Model file for the job. Use its own axes, mm. Give positions to 0.01 mm unless a question says otherwise; leave off trailing zeros. Order: outer loops, then holes, each group sorted by start corner. A loop starts at its lowest first (then second) coordinate and runs counter-clockwise, first axis right, second up. Notation, with made-up numbers: M 63,-33.5 L 108,-33.5 A25 ccw 108,-6.5 Z; hole C -7.5,73 d10. An arc over 180 degrees is marked long. Return JSON: item names as keys, results as strings. Group by question number.
1. Pin check, flat tip, straight feed: pin 1 (3 mm diameter, centred on x = -50, y = 50, fed in from +Z). Stop position of the tip, or through.
2. Slice it at B-B on z = -0.35. Give the number of separate pieces and of enclosed holes in the cut face, then the cut area to 3 significant figures.
3. Wall check: probe 1 along X at (y, z) = (-7, -0.2) (3 decimals); probe 2 along X at (y, z) = (-40, -0.9) (3 decimals); probe 3 along Y at (x, z) = (-50, -0.8) (3 decimals). Give the ranges that are in metal, low to high. Write a range as [from, to].
4. Slice it at A-A on y = 8.5. List the corners of the cut face in (x, z) (3 decimals), then the cut area to 4 significant figures.
from build123d import *

# Parameters (mm, degrees)
PAD_DEPTH        = 1
POCKET_DEPTH     = 0.001
HOLE_D           = 1.75
HOLE_CSINK_D     = 3.3
HOLE_CSINK_ANGLE = 90
SKETCH007_R      = 4.9
HOLE005_DEPTH    = 1.001
SKETCH008_R      = 1.5
HOLE006_DEPTH    = 1.001
SKETCH009_R      = 4.9
HOLE007_DEPTH    = 1.001
SKETCH010_R      = 1.5
HOLE008_DEPTH    = 1.001
POCKET001_DEPTH  = 1.001
SKETCH012_R      = 1.5
HOLE009_DEPTH    = 1.001


with BuildPart() as part:
    # Sketch → Pad (new body)
    with BuildSketch(Plane.XY):
        with BuildLine():
            Line((-51.8, 52.175), (51.8, 52.175))
            ThreePointArc((52.175, 51.8), (52.065165, 52.065165), (51.8, 52.175))
            Line((52.175, 51.8), (52.175, -51.8))
            ThreePointArc((51.8, -52.175), (52.065165, -52.065165), (52.175, -51.8))
            Line((51.8, -52.175), (-51.8, -52.175))
            ThreePointArc((-52.175, -51.8), (-52.065165, -52.065165), (-51.8, -52.175))
            Line((-52.175, -51.8), (-52.175, 51.8))
            ThreePointArc((-51.8, 52.175), (-52.065165, 52.065165), (-52.175, 51.8))
        make_face()
    extrude(amount=-PAD_DEPTH)

    # Sketch002 → Pocket (cut, through all)
    with BuildSketch(Plane.XY.offset(-4.8)):
        with BuildLine():
            Line((-45, 50.175), (45, 50.175))
            ThreePointArc((45, 50.175), (45.353553, 50.321447), (45.5, 50.675))
            ThreePointArc((45.5, 50.675), (45.353553, 51.028553), (45, 51.175))
            Line((-45, 51.175), (45, 51.175))
            ThreePointArc((-45, 51.175), (-45.353553, 51.028553), (-45.5, 50.675))
            ThreePointArc((-45.5, 50.675), (-45.353553, 50.321447), (-45, 50.175))
        make_face()
        with BuildLine():
            Line((-45, -51.175), (45, -51.175))
            ThreePointArc((45, -51.175), (45.353553, -51.028553), (45.5, -50.675))
            ThreePointArc((45.5, -50.675), (45.353553, -50.321447), (45, -50.175))
            Line((-45, -50.175), (45, -50.175))
            ThreePointArc((-45, -50.175), (-45.353553, -50.321447), (-45.5, -50.675))
            ThreePointArc((-45.5, -50.675), (-45.353553, -51.028553), (-45, -51.175))
        make_face()
        with BuildLine():
            Line((51.175, -45), (51.175, 45))
            ThreePointArc((51.175, 45), (51.028553, 45.353553), (50.675, 45.5))
            ThreePointArc((50.675, 45.5), (50.321447, 45.353553), (50.175, 45))
            Line((50.175, -45), (50.175, 45))
            ThreePointArc((50.175, -45), (50.321447, -45.353553), (50.675, -45.5))
            ThreePointArc((50.675, -45.5), (51.028553, -45.353553), (51.175, -45))
        make_face()
        with BuildLine():
            Line((-50.175, -45), (-50.175, 45))
            ThreePointArc((-50.175, 45), (-50.321447, 45.353553), (-50.675, 45.5))
            ThreePointArc((-50.675, 45.5), (-51.028553, 45.353553), (-51.175, 45))
            Line((-51.175, -45), (-51.175, 45))
            ThreePointArc((-51.175, -45), (-51.028553, -45.353553), (-50.675, -45.5))
            ThreePointArc((-50.675, -45.5), (-50.321447, -45.353553), (-50.175, -45))
        make_face()
    extrude(amount=-POCKET_DEPTH, mode=Mode.SUBTRACT)

    # Hole (through all)
    with Locations(Plane.XY):
        with Locations((-50, 50), (50, 50), (50, -50), (-50, -50)):
            CounterSinkHole(HOLE_D / 2, HOLE_CSINK_D / 2, counter_sink_angle=HOLE_CSINK_ANGLE)

    # Sketch007 → Hole005 (cut, through all)
    with BuildSketch(Plane.XY):
        with Locations((-40.005, -40.005)):
            Circle(SKETCH007_R)
        with Locations((-13.335, -40.005)):
            Circle(SKETCH007_R)
        with Locations((13.335, -40.005)):
            Circle(SKETCH007_R)
        with Locations((40.005, -40.005)):
            Circle(SKETCH007_R)
    extrude(amount=-HOLE005_DEPTH, mode=Mode.SUBTRACT)

    # Sketch008 → Hole006 (cut, through all)
    with BuildSketch(Plane.XY):
        with Locations((-40.005, -31.505)):
            Circle(SKETCH008_R)
        with Locations((-13.335, -31.505)):
            Circle(SKETCH008_R)
        with Locations((13.335, -31.505)):
            Circle(SKETCH008_R)
        with Locations((40.005, -31.505)):
            Circle(SKETCH008_R)
    extrude(amount=-HOLE006_DEPTH, mode=Mode.SUBTRACT)

    # Sketch009 → Hole007 (cut, through all)
    with BuildSketch(Plane.XY):
        with Locations((-40.005, 40.005)):
            Circle(SKETCH009_R)
        with Locations((-13.335, 40.005)):
            Circle(SKETCH009_R)
        with Locations((13.335, 40.005)):
            Circle(SKETCH009_R)
        with Locations((40.005, 40.005)):
            Circle(SKETCH009_R)
    extrude(amount=-HOLE007_DEPTH, mode=Mode.SUBTRACT)

    # Sketch010 → Hole008 (cut, through all)
    with BuildSketch(Plane.XY):
        with Locations((-40.005, 48.505)):
            Circle(SKETCH010_R)
        with Locations((-13.335, 48.505)):
            Circle(SKETCH010_R)
        with Locations((13.335, 48.505)):
            Circle(SKETCH010_R)
        with Locations((40.005, 48.505)):
            Circle(SKETCH010_R)
    extrude(amount=-HOLE008_DEPTH, mode=Mode.SUBTRACT)

    # Sketch011 → Pocket001 (cut, through all)
    with BuildSketch(Plane.XY):
        with BuildLine():
            ThreePointArc((-38.955, 18), (-40.005, 19.05), (-41.055, 18))
            Line((-41.055, 18), (-41.055, -18))
            ThreePointArc((-41.055, -18), (-40.005, -19.05), (-38.955, -18))
            Line((-38.955, 18), (-38.955, -18))
        make_face()
        with BuildLine():
            ThreePointArc((-12.285, 18), (-13.335, 19.05), (-14.385, 18))
            Line((-14.385, 18), (-14.385, -18))
            ThreePointArc((-14.385, -18), (-13.335, -19.05), (-12.285, -18))
            Line((-12.285, 18), (-12.285, -18))
        make_face()
        with BuildLine():
            ThreePointArc((14.385, 18), (13.335, 19.05), (12.285, 18))
            Line((12.285, 18), (12.285, -18))
            ThreePointArc((12.285, -18), (13.335, -19.05), (14.385, -18))
            Line((14.385, 18), (14.385, -18))
        make_face()
        with BuildLine():
            ThreePointArc((41.055, 18), (40.005, 19.05), (38.955, 18))
            Line((38.955, 18), (38.955, -18))
            ThreePointArc((38.955, -18), (40.005, -19.05), (41.055, -18))
            Line((41.055, 18), (41.055, -18))
        make_face()
    extrude(amount=-POCKET001_DEPTH, mode=Mode.SUBTRACT)

    # Sketch012 → Hole009 (cut, through all)
    with BuildSketch(Plane.XY):
        with Locations((-40.005, 25)):
            Circle(SKETCH012_R)
        with Locations((-13.335, 25)):
            Circle(SKETCH012_R)
        with Locations((13.335, 25)):
            Circle(SKETCH012_R)
        with Locations((40.005, 25)):
            Circle(SKETCH012_R)
    extrude(amount=-HOLE009_DEPTH, mode=Mode.SUBTRACT)


solid = part.part
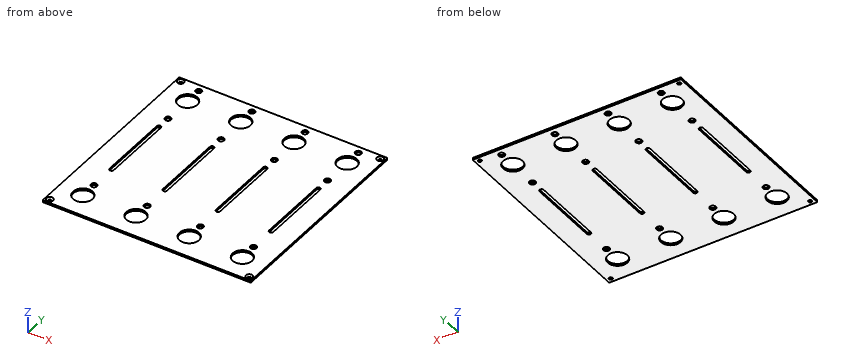
Result:
{
 "1": {"pin 1": "stops at z = -0.15"},
 "2": {"separate pieces": "1", "enclosed holes": "28", "area": "9,860 mm2"},
 "3": {"probe 1": "x = [-52.175, -41.055], [-38.955, -14.385], [-12.285, 12.285], [14.385, 38.955], [41.055, 52.175]", "probe 2": "x = [-52.175, -44.905], [-35.105, -18.235], [-8.435, 8.435], [18.235, 35.105], [44.905, 52.175]", "probe 3": "y = [-52.175, -50.875], [-49.125, 49.125], [50.875, 52.175]"},
 "4": {"outline": "M -52.175,-1 L -41.055,-1 L -41.055,0 L -52.175,0 Z; M -38.955,-1 L -14.385,-1 L -14.385,0 L -38.955,0 Z; M -12.285,-1 L 12.285,-1 L 12.285,0 L -12.285,0 Z; M 14.385,-1 L 38.955,-1 L 38.955,0 L 14.385,0 Z; M 41.055,-1 L 52.175,-1 L 52.175,0 L 41.055,0 Z", "area": "95.95 mm2"}
}
